Input: part model. Units: mm. Frame: model coordinates. A direction names the side the tool comes from. Round coordinates to 2 decimals unless told otherwise and drop trailing zeros. Write each loop counter-clockwise with the first axis right and the second up, starting at its lowest first coordinate (ties: lowest second). Pieces come first, ordered by that corner, then holes. Notation, with made-up numbers: (53.25, 62) -> (73.25, 62) arc R31 cw to (73.25, 98) -> close; hole circle Ø11 at (30, 84.25). An arc over 180 degrees is marked (long way). Write item = value, one per line.
```python
from build123d import *

# Parameters (mm, degrees)
SKETCH001_W  = 6
SKETCH001_H  = 6
PAD001_DEPTH = 0.1
FILLET001_R  = 0.3
PAD008_DEPTH = 0.7
FILLET003_R  = 0.29
PAD009_DEPTH = 0.7
FILLET004_R  = 0.29
PAD010_DEPTH = 0.7
FILLET005_R  = 0.29
SKETCH_W     = 6
SKETCH_H     = 6
PAD_DEPTH    = 3.5
FILLET_R     = 0.3
SKETCH004_R  = 0.5
PAD003_DEPTH = 0.6
SKETCH003_R  = 0.5
PAD004_DEPTH = 0.6
SKETCH005_R  = 0.5
PAD002_DEPTH = 0.6
SKETCH002_R  = 0.5
PAD005_DEPTH = 0.6
SKETCH006_R  = 1.75
PAD006_DEPTH = 4.5
FILLET006_R  = 0.1
PAD007_DEPTH = 0.7
FILLET002_R  = 0.29


with BuildPart() as fillet001:
    # Sketch001 → Pad001 (new body)
    with BuildSketch(Plane.XY.offset(3.5)):
        with Locations((3.15, -2.25)):
            Rectangle(SKETCH001_W, SKETCH001_H)
    extrude(amount=PAD001_DEPTH)

    # Fillet001
    fillet001_edges = [fillet001.edges().sort_by_distance(p)[0] for p in [
        (6.15, -5.25, 3.55),
        (0.15, -5.25, 3.55),
        (6.15, 0.75, 3.55),
        (0.15, 0.75, 3.55),
    ]]
    fillet(fillet001_edges, radius=FILLET001_R)


with BuildPart() as fillet003:
    # Sketch008 → Pad008 (new body)
    with BuildSketch(Plane.XZ.offset(0.35)):
        Polygon((-0.15, 1.5), (0.15, 1.5), (0.15, -0.5), (-0.15, -1.5), (0.15, -2.5), (0.15, -3.5), (-0.15, -3.5), (-0.15, -2.5), (-0.45, -1.5), (-0.15, -0.5), align=None)
    extrude(amount=-PAD008_DEPTH)

    # Fillet003
    fillet003_edges = [fillet003.edges().sort_by_distance(p)[0] for p in [
        (-0.15, 0, -2.5),
        (-0.15, 0, -0.5),
        (-0.45, 0, -1.5),
        (-0.15, 0, 1.5),
        (0.15, 0, -0.5),
        (-0.15, 0, -1.5),
        (0.15, 0, -2.5),
    ]]
    fillet(fillet003_edges, radius=FILLET003_R)


with BuildPart() as fillet004:
    # Sketch009 → Pad009 (new body)
    with BuildSketch(Plane.XZ.offset(4.85)):
        Polygon((6.45, 1.5), (6.15, 1.5), (6.15, -0.5), (6.45, -1.5), (6.15, -2.5), (6.15, -3.5), (6.45, -3.5), (6.45, -2.5), (6.75, -1.5), (6.45, -0.5), align=None)
    extrude(amount=-PAD009_DEPTH)

    # Fillet004
    fillet004_edges = [fillet004.edges().sort_by_distance(p)[0] for p in [
        (6.45, -4.5, -2.5),
        (6.45, -4.5, -0.5),
        (6.75, -4.5, -1.5),
        (6.45, -4.5, 1.5),
        (6.15, -4.5, -0.5),
        (6.45, -4.5, -1.5),
        (6.15, -4.5, -2.5),
    ]]
    fillet(fillet004_edges, radius=FILLET004_R)


with BuildPart() as fillet005:
    # Sketch010 → Pad010 (new body)
    with BuildSketch(Plane.XZ.offset(0.35)):
        Polygon((6.45, 1.5), (6.15, 1.5), (6.15, -0.5), (6.45, -1.5), (6.15, -2.5), (6.15, -3.5), (6.45, -3.5), (6.45, -2.5), (6.75, -1.5), (6.45, -0.5), align=None)
    extrude(amount=-PAD010_DEPTH)

    # Fillet005
    fillet005_edges = [fillet005.edges().sort_by_distance(p)[0] for p in [
        (6.45, 0, -2.5),
        (6.45, 0, -0.5),
        (6.75, 0, -1.5),
        (6.45, 0, 1.5),
        (6.15, 0, -0.5),
        (6.45, 0, -1.5),
        (6.15, 0, -2.5),
    ]]
    fillet(fillet005_edges, radius=FILLET005_R)


with BuildPart() as fillet_body:
    # Sketch → Pad (new body)
    with BuildSketch(Plane.XY):
        with Locations((3.15, -2.25)):
            Rectangle(SKETCH_W, SKETCH_H)
    extrude(amount=PAD_DEPTH)

    # Fillet
    fillet_edges = [fillet_body.edges().sort_by_distance(p)[0] for p in [
        (6.15, 0.75, 1.75),
        (6.15, -5.25, 1.75),
        (0.15, -5.25, 1.75),
        (0.15, 0.75, 1.75),
    ]]
    fillet(fillet_edges, radius=FILLET_R)


with BuildPart() as pad003:
    # Pad003 base: copy of Fillet body
    add(fillet_body.part)

    # Sketch004 → Pad003 (new body)
    with BuildSketch(Plane.XY.offset(3.5)):
        with Locations((5.15, -0.25)):
            Circle(SKETCH004_R)
    extrude(amount=PAD003_DEPTH)


with BuildPart() as pad004:
    # Pad004 base: copy of Fillet body
    add(fillet_body.part)

    # Sketch003 → Pad004 (new body)
    with BuildSketch(Plane.XY.offset(3.5)):
        with Locations((5.15, -4.25)):
            Circle(SKETCH003_R)
    extrude(amount=PAD004_DEPTH)


with BuildPart() as pad002:
    # Pad002 base: copy of Fillet body
    add(fillet_body.part)

    # Sketch005 → Pad002 (new body)
    with BuildSketch(Plane.XY.offset(3.5)):
        with Locations((1.15, -0.25)):
            Circle(SKETCH005_R)
    extrude(amount=PAD002_DEPTH)


with BuildPart() as pad005:
    # Pad005 base: copy of Fillet body
    add(fillet_body.part)

    # Sketch002 → Pad005 (new body)
    with BuildSketch(Plane.XY.offset(3.5)):
        with Locations((1.15, -4.25)):
            Circle(SKETCH002_R)
    extrude(amount=PAD005_DEPTH)


with BuildPart() as fillet006:
    # Pad006 base: copy of Fillet body
    add(fillet_body.part)

    # Sketch006 → Pad006 (new body)
    with BuildSketch(Plane.XY.offset(3.5)):
        with Locations((3.15, -2.25)):
            Circle(SKETCH006_R)
    extrude(amount=PAD006_DEPTH)

    # Fillet006
    fillet006_edges = [fillet006.edges().sort_by_distance(p)[0] for p in [
        (1.4, -2.25, 8),
    ]]
    fillet(fillet006_edges, radius=FILLET006_R)


with BuildPart() as obj1:
    # Sketch007 → Pad007 (new body)
    with BuildSketch(Plane.XZ.offset(4.85)):
        Polygon((-0.15, 1.5), (0.15, 1.5), (0.15, -0.5), (-0.15, -1.5), (0.15, -2.5), (0.15, -3.5), (-0.15, -3.5), (-0.15, -2.5), (-0.45, -1.5), (-0.15, -0.5), align=None)
    extrude(amount=-PAD007_DEPTH)

    # Fillet002
    fillet002_edges = [obj1.edges().sort_by_distance(p)[0] for p in [
        (-0.15, -4.5, -2.5),
        (-0.15, -4.5, -0.5),
        (-0.45, -4.5, -1.5),
        (-0.15, -4.5, 1.5),
        (0.15, -4.5, -0.5),
        (-0.15, -4.5, -1.5),
        (0.15, -4.5, -2.5),
    ]]
    fillet(fillet002_edges, radius=FILLET002_R)

    add(fillet001.part)
    add(fillet003.part)
    add(fillet004.part)
    add(fillet005.part)
    add(pad003.part)
    add(pad004.part)
    add(pad002.part)
    add(pad005.part)
    add(fillet006.part)


solid = obj1.part
```
1) Access query for faces 5 (the face through (5, 0, 4.1)), 6 (the face through (1, 0, 4.1)), 7 (the face through (1, -4, 4.1)), 8 (the face through (6.15, -2, 2)). Directions: +Z, -Z, +X, -X, +Y, -Y. A direction counts if a zero-diameter tool reaches every point of the face in a straight line with its end or side. Return the directions, or none.
Solutions:
face_5 = +Z, +X, +Y
face_6 = +Z, -X, +Y
face_7 = +Z, -X, -Y
face_8 = +Z, +X
2) Draft query along Y for faces 1 (the face through (5.627, -4.1, 3.846)), 2 (the face through (5, -4, 4.1)), 3 (the face through (3, -5.25, 2)), 4 (the face through (1.8, -0.9, 3.6)). Return one class per face: +Y half, -Y half, draft (parallel to the pull), parting line (faces both ways), or undercut.
Solutions:
face_1 = undercut
face_2 = draft
face_3 = -Y half
face_4 = undercut
3) Cut plane B-B (x = 3.15). Return the cut outline in (y, z), and give its area (3 significant figures).
Solutions:
outline = (-5.25, 0) -> (0.75, 0) -> (0.75, 3.6) -> (-0.5, 3.6) -> (-0.5, 7.9) arc R0.1 ccw to (-0.6, 8) -> (-3.9, 8) arc R0.1 ccw to (-4, 7.9) -> (-4, 3.6) -> (-5.25, 3.6) -> close
area = 37.0 mm^2
4) Cut plane D-D (x = 5.25). Return the cut outline in (y, z).
Solutions:
outline = (-5.25, 0) -> (0.75, 0) -> (0.75, 3.6) -> (0.24, 3.6) -> (0.24, 4.1) -> (-0.74, 4.1) -> (-0.74, 3.6) -> (-3.76, 3.6) -> (-3.76, 4.1) -> (-4.74, 4.1) -> (-4.74, 3.6) -> (-5.25, 3.6) -> close
5) Cut plane C-C (z = -1.75). Return the cut outline in (x, y) (3 decimals).
Solutions:
outline = (-0.375, -4.85) -> (-0.075, -4.85) -> (-0.075, -4.15) -> (-0.375, -4.15) -> close; (-0.375, -0.35) -> (-0.075, -0.35) -> (-0.075, 0.35) -> (-0.375, 0.35) -> close; (6.375, -4.85) -> (6.675, -4.85) -> (6.675, -4.15) -> (6.375, -4.15) -> close; (6.375, -0.35) -> (6.675, -0.35) -> (6.675, 0.35) -> (6.375, 0.35) -> close
6) First-contact query: P1, Ø0.8, axis at x = 5.5, y = 0, coming from the +Z side; P2, Ø1.8, axis at y = -3, z = 2, coming from the +X side; P3, Ø0.5, axis at y = -4.5, z = 0, coming from the -X side. Flat tips, straight axial feed; report the tip coordinate or a pass-through.
Solutions:
P1 = 4.1
P2 = 6.15
P3 = -0.15
7) Line query: L1, parallel to Y at x = 0, z = -2.25; L2, parallel to X at y = -0.25, z = 3.75; L3, parallel to Z at x = 0.75, y = -0.05. Output: solid intervals per line, ascending. Write a range as from..to.
Solutions:
L1 = -4.85..-4.15, -0.35..0.35
L2 = 0.65..1.65, 4.65..5.65
L3 = 0..4.1
8) Cut plane A-A (z = 2.5). Return the cut outline in (x, y).
Solutions:
outline = (0.15, -4.95) arc R0.3 ccw to (0.45, -5.25) -> (5.85, -5.25) arc R0.3 ccw to (6.15, -4.95) -> (6.15, 0.45) arc R0.3 ccw to (5.85, 0.75) -> (0.45, 0.75) arc R0.3 ccw to (0.15, 0.45) -> close
